```python
from build123d import *

# Parameters (mm, degrees)
SKETCH_1_W          = 12.5
SKETCH_1_H          = 10
EXTRUDE_1_DEPTH     = 3
SKETCH_2_R          = 0.85
SKETCH_2_R_2        = 2
CUT_EXTRUDE_1_DEPTH = 14.793114224
SKETCH_2_3_R        = 1.25
SKETCH_2_3_R_2      = 2
CUT_EXTRUDE_2_DEPTH = 1.5
SKETCH_3_W          = 9
SKETCH_3_H          = 10
EXTRUDE_2_DEPTH     = 30
EXTRUDE_2_2_DEPTH   = 30
SKETCH_3_3_W        = 3
SKETCH_3_3_H        = 10
EXTRUDE_3_DEPTH     = 3
SKETCH_3_4_W        = 6
SKETCH_3_4_H        = 10
SKETCH_3_4_R        = 2
SKETCH_3_4_R_2      = 1.25
CUT_EXTRUDE_3_DEPTH = 27
SKETCH_3_5_R        = 1.25
CUT_EXTRUDE_4_DEPTH = 38.245805133
CUT_EXTRUDE_START   = 27
SKETCH_3_6_R        = 2
SKETCH_3_6_R_2      = 1.25
CUT_EXTRUDE_5_DEPTH = 1.5


with BuildPart() as part:
    # Sketch 1 → Extrude 1 (new body)
    with BuildSketch(Plane.XY):
        with Locations((-6.25, 0)):
            Rectangle(SKETCH_1_W, SKETCH_1_H)
    extrude(amount=EXTRUDE_1_DEPTH)

    # Sketch 2 → Cut-Extrude 1 (cut, through all)
    with BuildSketch(Plane.XY.offset(3)):
        with Locations((-10.75, 0)):
            Circle(SKETCH_2_R)
        with Locations((-1.75, 0)):
            Circle(SKETCH_2_R)
        with Locations((-6.25, 0)):
            Circle(SKETCH_2_R_2)
    extrude(amount=-CUT_EXTRUDE_1_DEPTH, mode=Mode.SUBTRACT)

    # Sketch 2_3 → Cut-Extrude 2 (cut)
    with BuildSketch(Plane.XY.offset(3)):
        with Locations((-1.75, 0)):
            Circle(SKETCH_2_3_R)
        with Locations((-10.75, 0)):
            Circle(SKETCH_2_3_R)
        with Locations((-6.25, 0)):
            Circle(SKETCH_2_3_R_2)
    extrude(amount=-CUT_EXTRUDE_2_DEPTH, mode=Mode.SUBTRACT)



with BuildPart() as body_2:
    # Sketch 3 → Extrude 2 (new body)
    with BuildSketch(Plane(origin=(0, 0, 0), x_dir=(-1, 0, 0), z_dir=(0, 0, -1))):
        with Locations((-4.5, 0)):
            Rectangle(SKETCH_3_W, SKETCH_3_H)
    extrude(amount=EXTRUDE_2_DEPTH)


with BuildPart() as body_3:
    # Sketch 3 → Extrude 2 2 (new body)
    with BuildSketch(Plane(origin=(0, 0, 0), x_dir=(-1, 0, 0), z_dir=(0, 0, -1))):
        with Locations((17, 0)):
            Rectangle(SKETCH_3_W, SKETCH_3_H)
    extrude(amount=EXTRUDE_2_2_DEPTH)


with BuildPart() as part_1:
    add(part.part)

    add(body_2.part)  # Extrude 3 merges body 2

    add(body_3.part)  # Extrude 3 merges body 3
    # Sketch 3_3 → Extrude 3 (add)
    with BuildSketch(Plane(origin=(0, 0, 0), x_dir=(-1, 0, 0), z_dir=(0, 0, -1))):
        with Locations((14, 0)):
            Rectangle(SKETCH_3_3_W, SKETCH_3_3_H)
        with Locations((-1.5, 0)):
            Rectangle(SKETCH_3_3_W, SKETCH_3_3_H)
    extrude(amount=-EXTRUDE_3_DEPTH)

    # Sketch 3_4 → Cut-Extrude 3 (cut)
    # profile 1 of 6: a face of its own
    with BuildSketch(Plane(origin=(0, 0, 0), x_dir=(-1, 0, 0), z_dir=(0, 0, -1))):
        with Locations((-6, 0)):
            Rectangle(SKETCH_3_4_W, SKETCH_3_4_H)
        with Locations((-6, 0)):
            Circle(SKETCH_3_4_R, mode=Mode.SUBTRACT)
    # profile 2 of 6: a face of its own
    with BuildSketch(Plane(origin=(0, 0, 0), x_dir=(-1, 0, 0), z_dir=(0, 0, -1))):
        with Locations((18.5, 0)):
            Rectangle(SKETCH_3_4_W, SKETCH_3_4_H)
        with Locations((18.5, 0)):
            Circle(SKETCH_3_4_R, mode=Mode.SUBTRACT)
    # profile 3 of 6: a face of its own
    with BuildSketch(Plane(origin=(0, 0, 0), x_dir=(-1, 0, 0), z_dir=(0, 0, -1))):
        with Locations((-6, 0)):
            Circle(SKETCH_3_4_R)
        with Locations((-6, 0)):
            Circle(SKETCH_3_4_R_2, mode=Mode.SUBTRACT)
    # profile 4 of 6: a face of its own
    with BuildSketch(Plane(origin=(0, 0, 0), x_dir=(-1, 0, 0), z_dir=(0, 0, -1))):
        with Locations((-6, 0)):
            Circle(SKETCH_3_4_R_2)
    # profile 5 of 6: a face of its own
    with BuildSketch(Plane(origin=(0, 0, 0), x_dir=(-1, 0, 0), z_dir=(0, 0, -1))):
        with Locations((18.5, 0)):
            Circle(SKETCH_3_4_R)
        with Locations((18.5, 0)):
            Circle(SKETCH_3_4_R_2, mode=Mode.SUBTRACT)
    # profile 6 of 6: a face of its own
    with BuildSketch(Plane(origin=(0, 0, 0), x_dir=(-1, 0, 0), z_dir=(0, 0, -1))):
        with Locations((18.5, 0)):
            Circle(SKETCH_3_4_R_2)
    extrude(amount=CUT_EXTRUDE_3_DEPTH, mode=Mode.SUBTRACT)

    # Sketch 3_5 → Cut-Extrude 4 (cut, through all)
    with BuildSketch(Plane(origin=(0, 0, 0), x_dir=(-1, 0, 0), z_dir=(0, 0, -1))):
        with Locations(Location((18.5, 0, 0), (0, 0, 180))):
            Circle(SKETCH_3_5_R)
        with Locations(Location((-6, 0, 0), (0, 0, 180))):
            Circle(SKETCH_3_5_R)
    extrude(amount=CUT_EXTRUDE_4_DEPTH, mode=Mode.SUBTRACT)

    # Sketch 3_6 → Cut-Extrude 5 (cut)
    # profile 1 of 2: a face of its own
    with BuildSketch(Plane(origin=(0, 0, 0), x_dir=(-1, 0, 0), z_dir=(0, 0, -1)).offset(CUT_EXTRUDE_START)):
        with Locations(Location((18.5, 0, 0), (0, 0, 180))):
            Circle(SKETCH_3_6_R)
        with Locations(Location((18.5, 0, 0), (0, 0, 180))):
            Circle(SKETCH_3_6_R_2, mode=Mode.SUBTRACT)
    # profile 2 of 2: a face of its own
    with BuildSketch(Plane(origin=(0, 0, 0), x_dir=(-1, 0, 0), z_dir=(0, 0, -1)).offset(CUT_EXTRUDE_START)):
        with Locations(Location((-6, 0, 0), (0, 0, 180))):
            Circle(SKETCH_3_6_R)
        with Locations(Location((-6, 0, 0), (0, 0, 180))):
            Circle(SKETCH_3_6_R_2, mode=Mode.SUBTRACT)
    extrude(amount=CUT_EXTRUDE_5_DEPTH, mode=Mode.SUBTRACT)


solid = part_1.part
```
Could you check a few things on this model? Use its own coordinates, in mm. A direction names the side the tool comes from. Give positions to 0.01 mm unless a question says otherwise; leave off trailing zeros. Loops run counter-clockwise (first coordinate to the right, second up) from the corner with the lowest first, then second, coordinate; pieces in that order, holes last. Notation, with made-up numbers: (-20, 3.5) - (2, 3.5) arc R7 cw to (2, 14.5) - close; hole circle Ø6 at (26.25, 64). An arc over 180 degrees is marked (long way). Answer in a Markdown table with one row per item. Add a question column.
Q1. Which directions (+Z, -Z, +X, -X, +Y, -Y) give clear straight access to the entire face, cutting with the end or side of a thin tool? Please do faces 1 (the face through (4.75, -0.05, -29.24)), 2 (the face through (1, 5, -15)), 3 (the face through (-11, -1, 1.5)), 4 (the face through (-15.5, 0, -12)), 5 (the face through (0, 0, -15)).
Q2. If we section it at A-A (x = 6): List the corners of the cut face in (y, z) for me, plus the area to 4 significant figures.
Q3. If we section it at C-C (z = -12): List the corners of the cut face in (x, y) for me.
Q4. For pin 1 (3 mm diameter, centred on x = -10.5, y = -0.5, fed in from +Z); pin 2 (2 mm diameter, centred on x = -10.75, y = 0, fed in from +Z); pin 3 (2 mm diameter, centred on x = -10.75, y = 0, fed in from -Z); pin 4 (8 mm diameter, centred on x = -6, z = -20.5, fed in from -Y), each with a flat end and sliding along its axis, tell me the tip position at first contact or that it passes through.
Q5. Please list where these lines run through material, in increasing order: L1, parallel to Y at x = 6, z = -27.6; L2, parallel to X at y = -3.25, z = -3.5; L3, parallel to Y at x = -10.75, z = 1.9. Write a range as from..to.
Q6. We'd pull the mould along X, two halves only. Please class faces 6 (the face through (-17.345, 0.479, -29.24)), 7 (the face through (-21.5, 0, -28)), 8 (the face through (-16, 0, -27)), 9 (the face through (3, 0, -12)): +X half, -X half, draft (parallel to the pull), parting line (faces both ways), or undercut.
Q7. If we section it at D-D (x = -6.25): List the corners of the cut face in (y, z) for me, plus the area to 3 significant figures.
Q8. If we section it at B-B (y = 4): List the corners of the cut face in (x, z) for me, plus the area to 4 significant figures.
The answers:
| question | item | result |
|---|---|---|
| 1 | face 1 | +Z, -Z |
| 1 | face 2 | +Z, -Z, +X, -X, +Y |
| 1 | face 3 | +Z |
| 1 | face 4 | +Z, -X, +Y, -Y |
| 1 | face 5 | -Z, +Y, -Y |
| 2 | outline | (-5, -30) - (-1.25, -30) - (-1.25, -28.5) - (-2, -28.5) - (-2, -27) - (-5, -27) - close; (1.25, -30) - (5, -30) - (5, -27) - (2, -27) - (2, -28.5) - (1.25, -28.5) - close |
| 2 | area | 20.25 mm^2 |
| 3 | outline | (-15.5, -5) - (-12.5, -5) - (-12.5, 5) - (-15.5, 5) - close; (0, -5) - (3, -5) - (3, 5) - (0, 5) - close |
| 4 | pin 1 | stops at z = 3 |
| 4 | pin 2 | stops at z = 1.5 |
| 4 | pin 3 | stops at z = 0 |
| 4 | pin 4 | passes through |
| 5 | L1 | y = -5..-2, 2..5 |
| 5 | L2 | x = -15.5..-12.5, 0..3 |
| 5 | L3 | y = -5..-1.25, 1.25..5 |
| 6 | face 6 | undercut |
| 6 | face 7 | -X half |
| 6 | face 8 | draft |
| 6 | face 9 | +X half |
| 7 | outline | (-5, 0) - (-2, 0) - (-2, 3) - (-5, 3) - close; (2, 0) - (5, 0) - (5, 3) - (2, 3) - close |
| 7 | area | 18.0 mm^2 |
| 8 | outline | (-21.5, -30) - (-12.5, -30) - (-12.5, 0) - (0, 0) - (0, -30) - (9, -30) - (9, -27) - (3, -27) - (3, 3) - (-15.5, 3) - (-15.5, -27) - (-21.5, -27) - close |
| 8 | area | 271.5 mm^2 |
